Can you work these out from the drawing? Everything is in mm from the part's minimum corner. Round coordinates to 2 decimals unless told otherwise and drop trailing zeros. Write each loop counter-clockwise with the first axis right and the second up, starting at its lowest first coordinate (ties: lowest second). Pieces come first, ordered by that corner, then holes. Notation, with made-up numbers: (55.25, 35) - (94.25, 35) arc R20 cw to (94.25, 62) - close; hole circle Ø11 at (-6, -29.5). An arc over 180 degrees is marked (long way). One line per item, written item: value. Start each with the question number.
(1) If I drill on L1, parallel to Y at x = 6.5, z = 266.7; L2, parallel to Y at x = 6.5, z = 418; L3, parallel to Z at x = 12.25, y = 165, over which ranges is the centre line in solid material (lowest first)? Write a range as from..to.
(2) I want a section at A-A on x = 5.25. List the corners of the cut face in (y, z) for me.
(3) I'm going to push flat-ended pins straight in: pin 1 Ø4 at (x, z) = (4.5, 431.5) entering from -Y; pin 2 Ø1 at (x, y) = (9, 382) entering from +Z. Where does each tip first touch, or does it pass through?
(4) I want a section at B-B on y = 233. List the corners of the cut face in (x, z) for me.
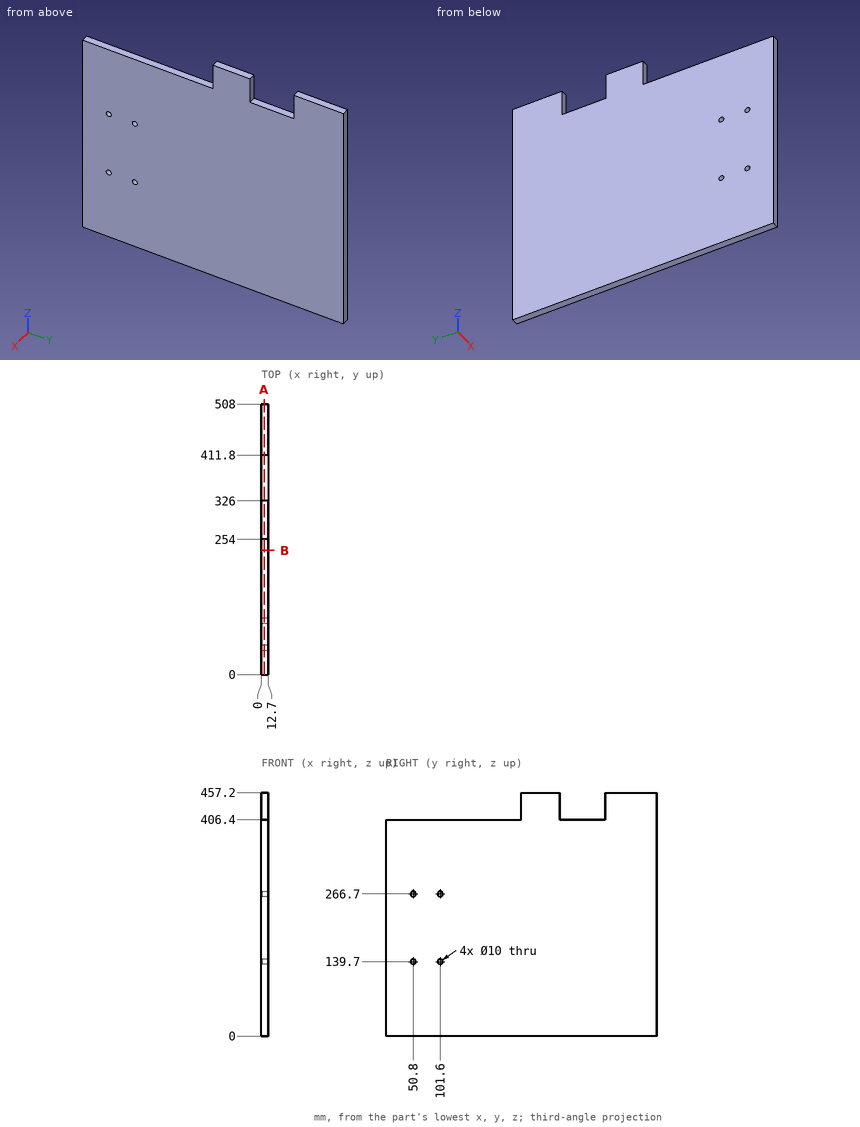
Established:
1. L1: 0..45.8, 55.8..96.6, 106.6..508
1. L2: 254..326, 411.8..508
1. L3: 0..406.4
2. outline: (0, 0) - (508, 0) - (508, 457.2) - (411.8, 457.2) - (411.8, 406.4) - (326, 406.4) - (326, 457.2) - (254, 457.2) - (254, 406.4) - (0, 406.4) - close; hole circle Ø10 at (50.8, 139.7); hole circle Ø10 at (50.8, 266.7); hole circle Ø10 at (101.6, 139.7); hole circle Ø10 at (101.6, 266.7)
3. pin 1: y = 254
3. pin 2: z = 406.4
4. outline: (0, 0) - (12.7, 0) - (12.7, 406.4) - (0, 406.4) - close
